```python
from build123d import *

# Parameters (mm, degrees)
F0_W     = 107.95
F0_H     = 31.75
F0_W_2   = 15.7988
F0_H_2   = 7.874
F0_R     = 10.16
F0_R_2   = 6.5024
F1_DEPTH = 3.175


with BuildPart() as f1:
    # F0 (on Top) → F1 (new body)
    with BuildSketch(Plane.XY):
        with Locations((-12.065, -3.762827)):
            Rectangle(F0_W, F0_H)
        with Locations((-51.8414, -4.524827)):
            Rectangle(F0_W_2, F0_H_2, mode=Mode.SUBTRACT)
        with Locations((-27.94, -3.762827)):
            Circle(F0_R, mode=Mode.SUBTRACT)
        with Locations((21.3106, -4.524827)):
            Rectangle(F0_W_2, F0_H_2, mode=Mode.SUBTRACT)
        with Locations((0, -3.762827)):
            Circle(F0_R_2, mode=Mode.SUBTRACT)
    extrude(amount=-F1_DEPTH)


solid = f1.part
```
Geometry check sheet. Reference: the model listing, model coordinates, mm. A direction names the side the tool comes from. Coordinates: 2 decimals unless noted, no trailing zeros. Loops run counter-clockwise (first coordinate to the right, second up) from the corner with the lowest first, then second, coordinate; pieces in that order, holes last.
Item 1: Sectioned sample at A-A, the plane x = 0. Record the boundary of the cut face in (y, z) (3 decimals), then the cut area to 3 significant figures.
Item 2: Sectioned sample at C-C, the plane z = -1.6. Record the boundary of the cut face in (x, y).
Item 3: Access from +Z, -Z, +X, -X, +Y, -Y to the whole of each face (thin tool, end or side, straight path). Record for faces 5 (the face through (-43.942, -5, -2)), 6 (the face through (-13, -4, 0)).
Item 4: Thickness scan on line 1 (Y direction, x = 0, z = -1.55); line 2 (Y direction, x = 16, z = -2.4); line 3 (X direction, y = -7.5, z = -2.15). Record the ranges inside material, lowest first.
Item 5: Release check for a two-part mould opening along X. For faces 1 (the face through (-13, -4, -3.175)), 2 (the face through (-52, -0.588, -2)), 3 (the face through (-66.04, -4, -2)), 4 (the face through (29.21, -5, -2)) record: released by +X, released by -X, zero draft, split by the parting line, or undercut.
Item 6: Go/stop test with flat-tipped pins: pin 1 Ø8 at (x, y) = (4, -9) entering from +Z; pin 2 Ø8 at (x, y) = (0, -3.76) entering from +Z. Record where each tip stops, or that it passes through.
Item 7: Sectioned sample at B-B, the plane y = 5. Record the boundary of the cut face in (x, z) (3 decimals), then the cut area to 3 significant figures.
Check result:
1. outline: (-19.638, -3.175) - (-10.265, -3.175) - (-10.265, 0) - (-19.638, 0) - close; (2.74, -3.175) - (12.112, -3.175) - (12.112, 0) - (2.74, 0) - close
1. area: 59.5 mm2
2. outline: (-66.04, -19.64) - (41.91, -19.64) - (41.91, 12.11) - (-66.04, 12.11) - close; hole (-59.74, -8.46) - (-43.94, -8.46) - (-43.94, -0.59) - (-59.74, -0.59) - close; hole circle Ø20.32 at (-27.94, -3.76); hole circle Ø13 at (0, -3.76); hole (13.41, -8.46) - (29.21, -8.46) - (29.21, -0.59) - (13.41, -0.59) - close
3. face 5: +Z, -Z
3. face 6: +Z, +X, -X, +Y, -Y
4. line 1: y = -19.64 to -10.27, 2.74 to 12.11
4. line 2: y = -19.64 to -8.46, -0.59 to 12.11
4. line 3: x = -66.04 to -59.74, -43.94 to -37.39, -18.49 to -5.32, 5.32 to 13.41, 29.21 to 41.91
5. face 1: zero draft
5. face 2: undercut
5. face 3: released by -X
5. face 4: undercut
6. pin 1: stops at z = 0
6. pin 2: passes through
7. outline: (-66.04, -3.175) - (-33.082, -3.175) - (-33.082, 0) - (-66.04, 0) - close; (-22.798, -3.175) - (41.91, -3.175) - (41.91, 0) - (-22.798, 0) - close
7. area: 310 mm2
